from build123d import *

# Parameters (mm, degrees)
F1_DEPTH = 75
F3_DEPTH = 200
F5_DEPTH = 100


with BuildPart() as f1:
    # F0 (on Front) → F1 (new body, symmetric)
    with BuildSketch(Plane.XZ):
        Polygon((85.300012, 25.884279), (0.300012, 25.884279), (-84.699988, 25.884279), (-84.699988, -4.115721), (-15.266005, -24.761366), (0.300012, 0.884279), (15.866029, -24.761366), (85.300012, -4.115721), align=None)
    extrude(amount=F1_DEPTH, both=True)

    # F2 (on face) → F3 (cut)
    with BuildSketch(Plane.XZ.offset(75)):
        Polygon((-17.53865, -18.869264), (0.300012, 10.520655), (18.138673, -18.869264), (80.300012, -0.386082), (80.300012, 20.884279), (-79.699988, 20.884279), (-79.699988, -0.386082), align=None)
    extrude(amount=-F3_DEPTH, mode=Mode.SUBTRACT)

    # F4 (on face) → F5 (intersect)
    with BuildSketch(Plane.XY.offset(25.884279)):
        with BuildLine():
            Line((92.307648, -27.267169), (99.30098, -26.961725))
            ThreePointArc((99.30098, -26.961725), (-3.949265, 68.282407), (-99.880233, -34.330005))
            Line((-99.880233, -34.330005), (-92.883447, -34.117915))
            ThreePointArc((-92.883447, -34.117915), (-3.690492, 61.287192), (92.307648, -27.267169))
        make_face()
    extrude(amount=-F5_DEPTH, mode=Mode.INTERSECT)


solid = f1.part
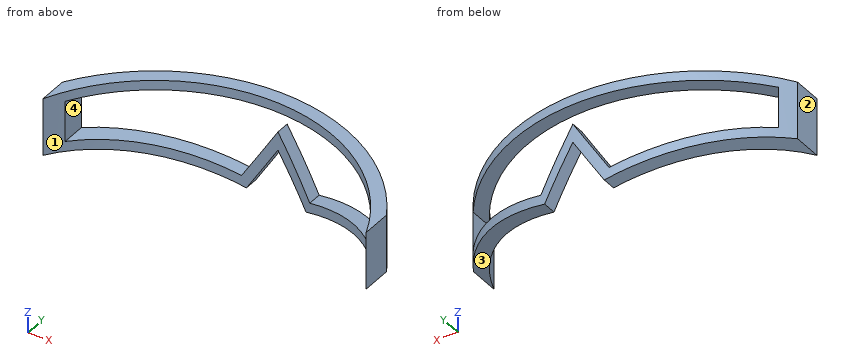
The listing builds one solid part. Answer for the finished solid, in the listing's coordinates (mm). Face numbers are marked on the shaded views. Give positions to 0.01 mm unless a question says otherwise; leave off trailing zeros. Write each loop counter-clockwise with the first axis right and the second up, starting at its lowest first coordinate (ties: lowest second). Pieces come first, ordered by that corner, then holes.
1) Given P1, Ø3.5, axis at y = 22.5, z = 6.5, coming from the +X side; P2, Ø1.5, axis at y = 29.5, z = 13, coming from the -X side, each flat-ended and moving along its own axis, determine where each tip first touches the part or whether it passes through.
2) Find the intervals of material crossed by L1, parallel to X at y = 65, z = -12.5; L2, parallel to X at y = 23, z = 14; L3, parallel to Z at x = 43.5, y = 58, in increasing order.
3) Section A-A (x = -4.5) is taken. Write down the section's boundary in (y, z), and give its area (3 significant figures).
4) For a pull along X with two mould halves and no side action, classify the marked faces 1, 2, 3 and 4 as pulls with the +X half, pulls with the -X half, needs draft (parallel to the pull), parting line crosses it, or undercut.
5) Section B-B (y = 57.5) is taken. Write down the section's boundary in (x, z).
6) Section C-C (z = -6.5) is taken. Write down the section's boundary in (x, y).
7) Section D-D (z = 4) is taken. Write down the section's boundary in (x, y), and give its area (3 significant figures).
Response:
1. P1: stops at x = 84.72
1. P2: stops at x = -79.8
2. L1: x = -13.67 to -7.82, 8.42 to 14.27
2. L2: x = -83.83 to -79.7, 80.3 to 83.3
2. L3: z = -16.54 to -11.33, 20.88 to 25.88
3. outline: (61.25, -7.02) - (68.26, -7.02) - (68.26, 2.61) - (61.25, 2.61) - close; (61.25, 20.88) - (68.26, 20.88) - (68.26, 25.88) - (61.25, 25.88) - close
3. area: 103 mm2
4. face 1: undercut
4. face 2: pulls with the -X half
4. face 3: pulls with the +X half
4. face 4: undercut
5. outline: (-45.49, -15.78) - (-26.7, -21.36) - (-26.7, -16.15) - (-45.49, -10.56) - close; (-45.49, 20.88) - (-26.7, 20.88) - (-26.7, 25.88) - (-45.49, 25.88) - close; (26.17, -21.7) - (44.96, -16.11) - (44.96, -10.9) - (26.17, -16.48) - close; (26.17, 20.88) - (44.96, 20.88) - (44.96, 25.88) - (26.17, 25.88) - close
6. outline: (-76.68, 21.1) arc R92.66 cw to (-59.14, 40.24) - (-59.14, 49.1) arc R99.66 ccw to (-76.68, 32.66) - close; (-10.03, 60.83) arc R92.66 cw to (-4.18, 61.27) - (-4.18, 68.27) arc R99.66 ccw to (-10.03, 67.87) - close; (4.78, 61.21) arc R92.66 cw to (10.63, 60.71) - (10.63, 67.75) arc R99.66 ccw to (4.78, 68.22) - close; (59.74, 39.3) arc R92.66 cw to (77.28, 19.41) - (77.28, 31.29) arc R99.66 ccw to (59.74, 48.26) - close
7. outline: (-84.7, 6.86) arc R92.66 cw to (-79.7, 16.4) - (-79.7, 28.88) arc R99.66 ccw to (-84.7, 21.63) - close; (-3.66, 61.29) arc R92.66 cw to (4.26, 61.24) - (4.26, 68.25) arc R99.66 ccw to (-3.66, 68.29) - close; (80.3, 14.46) arc R92.66 cw to (85.3, 4.25) - (85.3, 19.79) arc R99.66 ccw to (80.3, 27.35) - close
7. area: 193 mm2
